Model file for the job. Use its own axes, mm. A direction names the side the tool comes from. Round coordinates to 2 decimals unless told otherwise and drop trailing zeros. Write each loop counter-clockwise with the first axis right and the second up, starting at its lowest first coordinate (ties: lowest second). Pieces come first, ordered by that corner, then holes.
```python
from build123d import *

# Parameters (mm, degrees)
F3_R      = 24
F4_DEPTH  = 40
F0_R      = 15
F2_R      = 14.5
F7_DEPTH  = 40.0010001
F9_DEPTH  = 40
F10_W     = 38.0299583572
F10_H     = 24
F11_DEPTH = 85.7581399225
F12_R     = 10
F13_R     = 10


# Not quite as in the source:
# - a pattern or mirror of a feature is missing from the dataset's text; its kind, count and spacing are read off the source's solid


with BuildPart() as f4:
    # F3 (on Top) → F4 (new body)
    with BuildSketch(Plane.XY):
        Circle(F3_R)
    extrude(amount=-F4_DEPTH)

    # F0 (on Top) → F5 section 0
    with BuildSketch(Plane.XY):
        Circle(F0_R)
    # F2 (on offset) → F5 section 1
    with BuildSketch(Plane.XY.offset(-40)):
        Circle(F2_R)
    loft(mode=Mode.SUBTRACT)

    # F6 (on face) → F7 (cut, through all)
    with BuildSketch(Plane.XY):
        with BuildLine():
            Line((-13.6255430014, -6.272525641), (-13.6255430014, -19.7571399225))
            ThreePointArc((-13.6255430014, -19.7571399225), (0, -24), (13.6255430014, -19.7571399225))
            Line((13.6255430014, -19.7571399225), (13.6255430014, -6.272525641))
            ThreePointArc((13.6255430014, -6.272525641), (0, -15), (-13.6255430014, -6.272525641))
        make_face()
        with BuildLine():
            Line((-13.6255430014, -4.9592920782), (-13.6255430014, -6.272525641))
            ThreePointArc((-13.6255430014, -6.272525641), (0, -15), (13.6255430014, -6.272525641))
            Line((13.6255430014, -6.272525641), (13.6255430014, -4.9592920782))
            ThreePointArc((13.6255430014, -4.9592920782), (0, -14.5), (-13.6255430014, -4.9592920782))
        make_face()
    extrude(amount=-F7_DEPTH, mode=Mode.SUBTRACT)

    # F8 (on face) → F9 (join)
    with BuildSketch(Plane.XY):
        with BuildLine():
            Line((-13.6255430014, -61.7571399225), (-13.6255430014, -19.7571399225))
            ThreePointArc((-13.6255430014, -19.7571399225), (-21.248682689, -11.1576648087), (-24, 0))
            Line((-24, 0), (-59.6555013586, -61.7571399225))
            Line((-59.6555013586, -61.7571399225), (-13.6255430014, -61.7571399225))
        make_face()
        with BuildLine():
            ThreePointArc((24, 0), (21.248682689, -11.1576648087), (13.6255430014, -19.7571399225))
            Line((13.6255430014, -19.7571399225), (13.6255430014, -61.7571399225))
            Line((13.6255430014, -61.7571399225), (59.6555013586, -61.7571399225))
            Line((59.6555013586, -61.7571399225), (24, 0))
        make_face()
    extrude(amount=-F9_DEPTH)

    # F10 (on face) → F11 (cut, through all)
    with BuildSketch(Plane.XZ.offset(61.7571399225)):
        with Locations((-40.64052218, -20)):
            Rectangle(F10_W, F10_H)
    f11 = extrude(amount=-F11_DEPTH, mode=Mode.SUBTRACT)

    # F11_copies: F11 across plane
    add(f11.mirror(Plane(origin=(0, 0, 0), x_dir=(0, 0, 1), z_dir=(1, 0, 0))), mode=Mode.SUBTRACT)

    # F12
    f12_edges = [f4.edges().sort_by_distance(p)[0] for p in [
        (-59.655501, -61.75714, -4),
        (-59.655501, -61.75714, -36),
        (-24, 0, -4),
        (-24, 0, -36),
    ]]
    fillet(f12_edges, radius=F12_R)

    # F13
    f13_edges = [f4.edges().sort_by_distance(p)[0] for p in [
        (59.655501, -61.75714, -4),
        (59.655501, -61.75714, -36),
        (24, 0, -4),
        (24, 0, -36),
    ]]
    fillet(f13_edges, radius=F13_R)


solid = f4.part
```
1) Wall check: probe 1 along X at (y, z) = (-14, -30.5); probe 2 along Z at (x, y) = (26, -47.5); probe 3 along X at (y, z) = (-26, -7). Give the ranges that are in metal, low to high.
2) Cut at C-C on z = -18. List the corners of the cut face in (x, y) (3 decimals), and give its area (3 significant figures).
3) Which spindle directions (+Z, -Z, +X, -X, +Y, -Y) get a long thin tool onto all of the face, cutting with end or side? Do faces 1 (the face through (-37.925, -24.119, -35.944)), 2 (the face through (21.626, -26, -20)), 3 (the face through (-34, -42, -8)), 4 (the face through (-13.626, -34, -20)). Say none if no direction does.
4) Cut at D-D on x = 44.5. List the corners of the cut face in (y, z).
5) Pull direction Z, two halves, no side cores. Call faces 5 (the face through (34, -42, -32)), 6 (the face through (51.068, -56.63, -4.056)), 7 (the face through (-34, -42, -32)), 8 (the face through (23, -28, -40)): released by +Z, released by -Z, zero draft, split by the parting line, or undercut.
6) Flat gauge pins, fed straight in: pin 1 Ø1 at (y, z) = (4, -30.5) entering from -X; pin 2 Ø15.5 at (x, y) = (39, -8.5) entering from -Z; pin 3 Ø10 at (y, z) = (-2.5, -12.5) entering from +X; pin 4 Ø2 at (y, z) = (-47.5, -16) entering from +X. Where does each tip first touch, or does it go through?
7) Cut at B-B on x = -43.5. List the corners of the cut face in (y, z) (3 decimals).
8) Cut at A-A on y = -33. List the corners of the cut face in (x, z), and give its area (3 significant figures).
Result sheet:
1. probe 1: x = -21.63 to -13.63, 13.63 to 21.63
1. probe 2: z = -40 to -32, -8 to 0
1. probe 3: x = -39.01 to -13.63, 13.63 to 39.01
2. outline: (-21.626, -61.757) - (-13.626, -61.757) - (-13.626, -5.714) arc R14.775 cw (long way) to (13.626, -5.714) - (13.626, -61.757) - (21.626, -61.757) - (21.626, 10.408) arc R24 ccw to (-21.626, 10.408) - close
2. area: 1,510 mm2
3. face 1: +Z, -Z, -X, +Y
3. face 2: +X, +Y, -Y
3. face 3: -X, +Y, -Y
3. face 4: +Z, -Z, -Y
4. outline: (-61.52, -40) - (-35.51, -40) - (-35.51, -32) - (-61.52, -32) - close; (-61.52, -8) - (-35.51, -8) - (-35.51, 0) - (-61.52, 0) - close
5. face 5: undercut
5. face 6: zero draft
5. face 7: undercut
5. face 8: released by -Z
6. pin 1: stops at x = -21.63
6. pin 2: passes through
6. pin 3: stops at x = 26.7
6. pin 4: stops at x = 21.63
7. outline: (-61.689, -40) - (-33.775, -40) - (-33.775, -32) - (-61.689, -32) - close; (-61.689, -8) - (-33.775, -8) - (-33.775, 0) - (-61.689, 0) - close
8. outline: (-43.05, -40) - (-13.63, -40) - (-13.63, 0) - (-43.05, 0) - (-43.05, -8) - (-21.63, -8) - (-21.63, -32) - (-43.05, -32) - close; (13.63, -40) - (43.05, -40) - (43.05, -32) - (21.63, -32) - (21.63, -8) - (43.05, -8) - (43.05, 0) - (13.63, 0) - close
8. area: 1,330 mm2
